Geometry check sheet. Reference: the model listing, model coordinates, mm. Face numbers are marked on the shaded views. A direction names the side the tool comes from. Coordinates: 2 decimals unless noted, no trailing zeros. Loops run counter-clockwise (first coordinate to the right, second up) from the corner with the lowest first, then second, coordinate; pieces in that order, holes last. Notation, with made-up numbers: (38, 71.25) - (72, 71.25) arc R29 ccw to (72, 91.25) - close; hole circle Ø6 at (57, -17.5). An arc over 180 degrees is marked (long way). One line per item, written item: value.
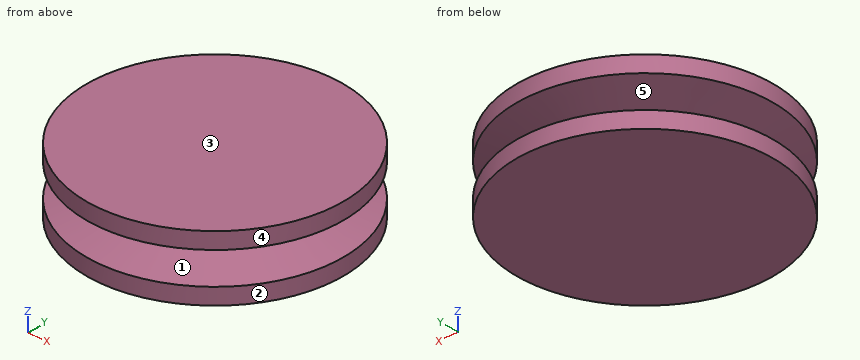
Autodesk Inventor part; units mm, degrees
ref_plane "Плоскость ремня" through (0, 13.8, 5) normal (0, 0, 1) x (1, 0, 0)
ref_plane "YZ Plane" through (0, 0, 0) normal (1, 0, 0) x (0, 1, 0)
ref_plane "XZ Plane" through (0, 0, 0) normal (0, 1, 0) x (-1, 0, 0)
sketch "Основной эскиз" plane through (0, 0, 0) normal (1, 0, 0) x (0, 1, 0)
  line L0 (0, 10) -> (19.8, 10)
  line L1 (19.8, 10) -> (19.8, 7.4728)
  line L2 (19.8, 7.4728) -> (13.8, 5.7523)
  line L3 (13.8, 5.7523) -> (13.8, 4.2477)
  line L4 (13.8, 4.2477) -> (19.8, 2.5272)
  line L5 (19.8, 2.5272) -> (19.8, 0)
  line L6 (19.8, 0) -> (0, 0)
  line L7 (18.5, 7.1) -> (18.5, 2.9) construction
  line L8 (13.8, 5) -> (18.5, 5) construction
  line L9 (19.8, 7.4728) -> (19.8, 2.5272)
  line L10 (0, -2) -> (0, 12)
  line L11 (0, 0) -> (0, 10)
  dimension "d0" = 4.2
  dimension "d1" = 32
  dimension "d2" = 1.3
  dimension "d6" = 10
  dimension "d21" = 37
  dimension "d25" = 6
  dimension "d27" = 5
ref_plane "Плоскость ремня" through (0, 13.8, 5) normal (0, 0, 1) x (1, 0, 0)
revolve "Тело" add sketch "Основной эскиз" angle 360 about axis through (0, 0, -10) along (0, 0, 1)
revolve "Канавка" cut sketch "Основной эскиз" angle 360 about axis through (0, 0, -10) along (0, 0, 1) contours L9 L4 L3 L2
fillet "Сопряжение снаружи" [suppressed]
fillet "Сопряжение изнутри" [suppressed]
pattern_of_one "Образец канавки"
equation "\"d0\" = da_Bw"
equation "\"d1\" = da_Alfa"
equation "\"d2\" = da_c"
equation "\"d21\" = da_Dw"
equation "\"d25\" = da_Hd"
equation "\"d27\" = da_Se"
equation "\"da_r1\" = 0"
equation "\"da_r2\" = 0"
equation "\"d18\" = da_Sg"
equation "\"d5\" = da_Se"
equation "\"da_Bw\" = 4.2"
equation "\"da_Alfa\" = 32deg"
equation "\"da_c\" = 1.3"
equation "\"da_Dw\" = 37"
equation "\"da_Hd\" = 6"
equation "\"da_Se\" = 5"
equation "\"da_Sg\" = 6"
properties part number "Шкив желобчатый2" material "Steel"
(1) Cross-section at A-A on x = 0. Record the cut outline in (y, z), and give its area (3 significant figures).
Reply:
outline: (-19.8, 0) - (19.8, 0) - (19.8, 2.53) - (13.8, 4.25) - (13.8, 5.75) - (19.8, 7.47) - (19.8, 10) - (-19.8, 10) - (-19.8, 7.47) - (-13.8, 5.75) - (-13.8, 4.25) - (-19.8, 2.53) - close
area: 357 mm2
(2) Cross-section at D-D on z = 8. Record the cut outline in (x, y), and give its area (3 significant figures).
Reply:
outline: circle Ø39.6 at (0, 0)
area: 1,230 mm2
(3) Cross-section at C-C on z = 5. Record the cut outline in (x, y).
Reply:
outline: circle Ø27.6 at (0, 0)
(4) Material ranges on probe 1 along Z at (x, y) = (-17, 4); probe 2 along Z at (x, y) = (-15, 1); probe 3 along X at (y, z) = (11.5, 5), recorded low to high. Write a range as from..to.
Reply:
probe 1: 0..3.2, 6.8..10
probe 2: 0..3.89, 6.11..10
probe 3: -7.63..7.63
(5) Release check for a two-part mould opening along Z. For the marked faces 3, 4 and 5 record: pulls with the +Z half, pulls with the -Z half, needs draft (parallel to the pull), parting line crosses it, or undercut.
Reply:
face 3: pulls with the +Z half
face 4: needs draft
face 5: undercut
(6) Access from +Z, -Z, +X, -X, +Y, -Y to the whole of each face (thin tool, end or side, straight path). Record for the marked faces 1 and 2.
Reply:
face 1: none
face 2: +Z, -Z
(7) Go/stop test with flat-tipped pins: pin 1 Ø4 at (y, z) = (2.5, 8.5) entering from -X; pin 2 Ø3 at (y, z) = (6.5, 2) entering from -X; pin 3 Ø2 at (y, z) = (13, 1) entering from -X. Record where each tip stops, or that it passes through.
Reply:
pin 1: x = -19.79
pin 2: x = -19.16
pin 3: x = -15.75
